from build123d import *

# Parameters (mm, degrees)
BOSS_EXTRUDE1_DEPTH = 2.54
FILLET1_R           = 1.27


with BuildPart() as part:
    # Sketch1 → Boss-Extrude1 (new body)
    with BuildSketch(Plane(origin=(0, 0, 0), x_dir=(1, 0, 0), z_dir=(0, 1, 0))):
        Polygon((0, 0), (0, 31.75), (3.175, 31.75), (3.175, 38.1), (41.275, 12.7), (41.275, -6.35), (3.175, -6.35), (3.175, 0), align=None)
    extrude(amount=BOSS_EXTRUDE1_DEPTH)

    # Fillet1
    fillet1_edges = [part.edges().sort_by_distance(p)[0] for p in [
        (41.275, 0, -3.175),
        (22.225, 0, 6.35),
        (22.225, 2.54, 6.35),
        (3.175, 1.27, -38.1),
        (41.275, 1.27, -12.7),
        (41.275, 1.27, 6.35),
        (3.175, 1.27, 6.35),
        (41.275, 2.54, -3.175),
        (22.225, 2.54, -25.4),
        (22.225, 0, -25.4),
    ]]
    fillet(fillet1_edges, radius=FILLET1_R - 0.0001)  # a hair under: the kernel refuses the full size


solid = part.part
Work out the finished part from the listing and answer in its coordinate system (mm). A direction names the side the tool comes from. Coordinates: 2 decimals unless noted, no trailing zeros. Loops run counter-clockwise (first coordinate to the right, second up) from the corner with the lowest first, then second, coordinate; pieces in that order, holes last. Notation, with made-up numbers: M -26.75,-5.75 L 31.25,-5.75 A20 ccw 31.25,24.25 Z; hole C 56.25,59 d3. An arc over 180 degrees is marked long. Answer in a Markdown table with one row per item. Add a question column.
1. A flat-ended cylindrical pin translates along its axis: P1, Ø0.8, axis at x = 1, y = 1.5, coming from the +Z side. Find the tip coordinate at first contact, or state that the pin passes through.
2. A tool of negligible diameter and unlimited length cuts with its end or side. For faces 1 (the cylindrical face through (40.91, 2.16, -3.35)), 2 (the flat face through (2, 1, 0)), 3 (the flat face through (2, 1, -31.75)), from which of +Z, -Z, +X, -X, +Y, -Y can it reach the whole face along a straight path? Write none if from no direction.
3. Find section B-B, the plane y = 2. Write down the section's boundary in (x, z) (3 decimals), then the cut area to 3 significant figures.
4. Consider L1, parallel to Z at x = 21, y = 0.75; L2, parallel to Z at x = 22.5, y = 1.35; L3, parallel to X at y = 1.1, z = -25. Determine where each line is inside the solid, lowest interval first.
Reported:
| question | item | result |
|---|---|---|
| 1 | P1 | stops at z = 0 |
| 2 | face 1 | +Z, -Z, +X, +Y |
| 2 | face 2 | +Z, -X, +Y, -Y |
| 2 | face 3 | -Z, -X, +Y, -Y |
| 3 | outline | M 0,-31.75 L 3.175,-31.75 L 3.175,-35.727 A1.27 ccw 4.414,-36.997 L 40.582,-12.885 A1.039 ccw 41.044,-12.02 L 41.044,5.08 A1.039 ccw 40.005,6.119 L 3.715,6.119 A1.27 ccw 3.175,5.08 L 3.175,0 L 0,0 Z |
| 3 | area | 1,290 mm^2 |
| 4 | L1 | z = -26.08 to 6.24 |
| 4 | L2 | z = -25.21 to 6.35 |
| 4 | L3 | x = 0 to 22.8 |
